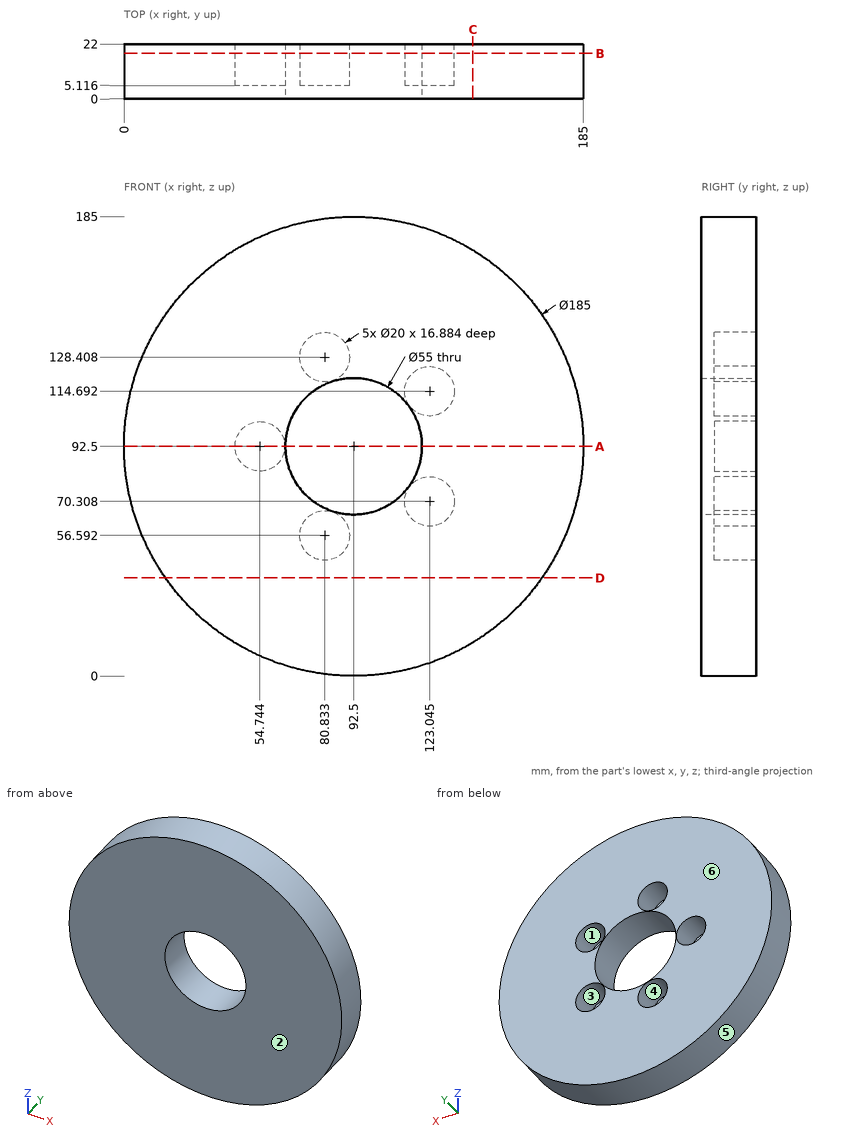
Design review of the part shown in the three views and the two pictorial views. Dimensions are in mm from the part's minimum x, y and z. A direction names the side the tool comes from. Give positions to 0.01 mm unless a question says otherwise; leave off trailing zeros. Loops run counter-clockwise (first coordinate to the right, second up) from the corner with the lowest first, then second, coordinate; pieces in that order, holes last. Notation, with made-up numbers: M 53,11.25 L 89,11.25 A27 ccw 89,27.25 Z; hole C 25,-1 d3. An arc over 180 degrees is marked long. Answer as a JSON object with one key per item and string values. Group by question number.
Q1. Add section A-A on z = 92.5. Give the boundary of the cut face in (x, y), and give its area (3 significant figures).
Q2. Insertion check: P1, Ø2, axis at x = 55, y = 19, coming from the -Z side (1 decimal); P2, Ø16, axis at x = 80.83, z = 128.41, coming from the +Y side; P3, Ø3, axis at x = 30, y = 17.5, coming from the +Z side (1 decimal). Each pin has a flat end and moves straight along its axis. Give the tip position at first contact, or say it passes through.
Q3. Mouldability with a two-part tool opening along X and no side actions: class the marked faces 3, 4, 5 and 6 as +X half, -X half, draft (parallel to the pull), parting line (faces both ways), or undercut.
Q4. Add section C-C on x = 140.5. Give the boundary of the cut face in (y, z), and give its area (3 significant figures).
Q5. For probe 1 along X at (y, z) = (12.5, 92.5); probe 2 along Z at (x, y) = (80.5, 9) (1 decimal); probe 3 along X at (y, z) = (4.5, 94), list the stretches that pass through material, from the lowest coordinate up. Write a range as [from, to].
Q6. Add section D-D on z = 39.5. Give the boundary of the cut face in (x, y).
Q7. Add section B-B on y = 18.25. Give the boundary of the cut face in (x, z) (1 decimal).
Q8. Tool access review of the marked faces 1 and 2: name each direction out of +Z, -Z, +X, -X, +Y, -Y from which nothing blocks a thin tool from reaching the whole face with its end or side.
Checked values:
{
 "1": {"outline": "M 0,0 L 65,0 L 65,22 L 64.74,22 L 64.74,5.12 L 44.74,5.12 L 44.74,22 L 0,22 Z; M 120,0 L 185,0 L 185,22 L 120,22 Z", "area": "2,520 mm²"},
 "2": {"P1": "z = 7.5", "P2": "y = 5.12", "P3": "z = 162"},
 "3": {"face 3": "undercut", "face 4": "undercut", "face 5": "parting line", "face 6": "draft"},
 "4": {"outline": "M 0,13.43 L 22,13.43 L 22,171.57 L 0,171.57 Z", "area": "3,480 mm²"},
 "5": {"probe 1": "[0, 44.74], [64.74, 65], [120, 185]", "probe 2": "[0.8, 46.6], [66.6, 67.8], [117.2, 118.4], [138.4, 184.2]", "probe 3": "[0.01, 65.04], [119.96, 184.99]"},
 "6": {"outline": "M 16.69,0 L 168.31,0 L 168.31,22 L 16.69,22 Z"},
 "7": {"outline": "C 92.5,92.5 d185; hole C 54.7,92.5 d20; hole C 92.5,92.5 d55; hole C 80.8,56.6 d20; hole C 80.8,128.4 d20; hole C 123,70.3 d20; hole C 123,114.7 d20"},
 "8": {"face 1": "+Y", "face 2": "+Z, -Z, +X, -X, -Y"}
}
